from build123d import *

# Parameters (mm, degrees)
SKETCH_1_W          = 720
SKETCH_1_H          = 600
EXTRUDE_1_DEPTH     = 10
CUT_EXTRUDE_2_DEPTH = 469.72166581


with BuildPart() as part:
    # 草圖1 → 填料-伸長1 (new body)
    with BuildSketch(Plane.XY):
        Rectangle(SKETCH_1_W, SKETCH_1_H)
    extrude(amount=EXTRUDE_1_DEPTH)

    # 草圖2 → 除料-伸長2 (cut, through all)
    with BuildSketch(Plane.XY.offset(10)):
        with BuildLine():
            Line((-227, -52), (-195.192212959, -52))
            ThreePointArc((-195.192212959, -52), (-195.455703203, -51.000667501), (-195.714077164, -50))
            Line((-195.714077164, -50), (-225, -50))
            Line((-225, -50), (-225, 50))
            Line((-225, 50), (-195.714077164, 50))
            ThreePointArc((-195.714077164, 50), (-195.455703203, 51.000667501), (-195.192212959, 52))
            Line((-195.192212959, 52), (-227, 52))
            Line((-227, 52), (-227, -52))
        make_face()
        with BuildLine():
            Line((-225, -50), (-195.714077164, -50))
            ThreePointArc((-195.714077164, -50), (-202, 0), (-195.714077164, 50))
            Line((-195.714077164, 50), (-225, 50))
            Line((-225, 50), (-225, -50))
        make_face()
        with BuildLine():
            ThreePointArc((-193.64916731, 50), (-200, 0), (-193.64916731, -50))
            Line((-193.64916731, -50), (-125, -50))
            Line((-125, -50), (-125, 50))
            Line((-125, 50), (-193.64916731, 50))
        make_face()
        with BuildLine():
            ThreePointArc((-195.714077164, 50), (-202, 0), (-195.714077164, -50))
            Line((-195.714077164, -50), (-193.64916731, -50))
            ThreePointArc((-193.64916731, -50), (-200, 0), (-193.64916731, 50))
            Line((-193.64916731, 50), (-195.714077164, 50))
        make_face()
        with BuildLine():
            ThreePointArc((-193.64916731, 50), (-193.388030784, 51.000681851), (-193.121723273, 52))
            Line((-193.121723273, 52), (-195.192212959, 52))
            ThreePointArc((-195.192212959, 52), (-195.455703203, 51.000667501), (-195.714077164, 50))
            Line((-195.714077164, 50), (-193.64916731, 50))
        make_face()
        with BuildLine():
            ThreePointArc((-193.121723273, 52), (-141.421356237, 141.421356237), (-52, 193.121723273))
            Line((-52, 193.121723273), (-52, 195.192212959))
            ThreePointArc((-52, 195.192212959), (-142.8355698, 142.8355698), (-195.192212959, 52))
            Line((-195.192212959, 52), (-193.121723273, 52))
        make_face()
        with BuildLine():
            ThreePointArc((134.208828858, -148.283479378), (170.598797446, -104.384147791), (193.121723273, -52))
            Line((193.121723273, -52), (123, -52))
            Line((123, -52), (123, 52))
            Line((123, 52), (193.121723273, 52))
            ThreePointArc((193.121723273, 52), (141.421356237, 141.421356237), (52, 193.121723273))
            Line((52, 193.121723273), (52, 98))
            Line((52, 98), (-52, 98))
            Line((-52, 98), (-52, 193.121723273))
            ThreePointArc((-52, 193.121723273), (-141.421356237, 141.421356237), (-193.121723273, 52))
            Line((-193.121723273, 52), (-123, 52))
            Line((-123, 52), (-123, -52))
            Line((-123, -52), (-193.121723273, -52))
            ThreePointArc((-193.121723273, -52), (-170.598797446, -104.384147791), (-134.208828858, -148.283479378))
            Line((-134.208828858, -148.283479378), (-50, -224.499443206))
            ThreePointArc((-50, -224.499443206), (0, -230), (50, -224.499443206))
            Line((50, -224.499443206), (134.208828858, -148.283479378))
        make_face()
        with BuildLine():
            ThreePointArc((-193.64916731, -50), (-193.388030784, -51.000681851), (-193.121723273, -52))
            Line((-193.121723273, -52), (-123, -52))
            Line((-123, -52), (-123, 52))
            Line((-123, 52), (-193.121723273, 52))
            ThreePointArc((-193.121723273, 52), (-193.388030784, 51.000681851), (-193.64916731, 50))
            Line((-193.64916731, 50), (-125, 50))
            Line((-125, 50), (-125, -50))
            Line((-125, -50), (-193.64916731, -50))
        make_face()
        with BuildLine():
            Line((50, 100), (50, 193.64916731))
            ThreePointArc((50, 193.64916731), (25.200858902, 198.405939202), (8.18e-07, 200))
            ThreePointArc((8.18e-07, 200), (-25.200858091, 198.405939305), (-50, 193.64916731))
            Line((-50, 193.64916731), (-50, 100))
            Line((-50, 100), (50, 100))
        make_face()
        with BuildLine():
            Line((52, 98), (52, 193.121723273))
            ThreePointArc((52, 193.121723273), (51.000681851, 193.388030784), (50, 193.64916731))
            Line((50, 193.64916731), (50, 100))
            Line((50, 100), (-50, 100))
            Line((-50, 100), (-50, 193.64916731))
            ThreePointArc((-50, 193.64916731), (-51.000681851, 193.388030784), (-52, 193.121723273))
            Line((-52, 193.121723273), (-52, 98))
            Line((-52, 98), (52, 98))
        make_face()
        with BuildLine():
            ThreePointArc((-50, 195.714077164), (-39.236011871, 198.152808137), (-28.354893758, 200))
            Line((-28.354893758, 200), (-50, 200))
            Line((-50, 200), (-50, 195.714077164))
        make_face()
        with BuildLine():
            ThreePointArc((-28.354893758, 200), (-14.212670404, 201.499379652), (0, 202))
            Line((0, 202), (-52, 202))
            Line((-52, 202), (-52, 195.192212959))
            ThreePointArc((-52, 195.192212959), (-51.000667501, 195.455703203), (-50, 195.714077164))
            Line((-50, 195.714077164), (-50, 200))
            Line((-50, 200), (-28.354893758, 200))
        make_face()
        with BuildLine():
            Line((-52, 195.192212959), (-52, 193.121723273))
            ThreePointArc((-52, 193.121723273), (-51.000681851, 193.388030784), (-50, 193.64916731))
            Line((-50, 193.64916731), (-50, 195.714077164))
            ThreePointArc((-50, 195.714077164), (-51.000667501, 195.455703203), (-52, 195.192212959))
        make_face()
        with BuildLine():
            ThreePointArc((-50, 193.64916731), (-25.200858091, 198.405939305), (8.18e-07, 200))
            Line((8.18e-07, 200), (-28.354893758, 200))
            ThreePointArc((-28.354893758, 200), (-39.236011871, 198.152808137), (-50, 195.714077164))
            Line((-50, 195.714077164), (-50, 193.64916731))
        make_face()
        with BuildLine():
            ThreePointArc((28.354893758, 200), (14.212670404, 201.499379652), (0, 202))
            ThreePointArc((0, 202), (-14.212670404, 201.499379652), (-28.354893758, 200))
            Line((-28.354893758, 200), (8.18e-07, 200))
            Line((8.18e-07, 200), (28.354893758, 200))
        make_face()
        with BuildLine():
            ThreePointArc((50, 195.714077164), (51.000667501, 195.455703203), (52, 195.192212959))
            Line((52, 195.192212959), (52, 202))
            Line((52, 202), (0, 202))
            ThreePointArc((0, 202), (14.212670404, 201.499379652), (28.354893758, 200))
            Line((28.354893758, 200), (50, 200))
            Line((50, 200), (50, 195.714077164))
        make_face()
        with BuildLine():
            Line((50, 193.64916731), (50, 195.714077164))
            ThreePointArc((50, 195.714077164), (39.236011871, 198.152808137), (28.354893758, 200))
            Line((28.354893758, 200), (8.18e-07, 200))
            ThreePointArc((8.18e-07, 200), (25.200858902, 198.405939202), (50, 193.64916731))
        make_face()
        with BuildLine():
            ThreePointArc((28.354893758, 200), (39.236011871, 198.152808137), (50, 195.714077164))
            Line((50, 195.714077164), (50, 200))
            Line((50, 200), (28.354893758, 200))
        make_face()
        with BuildLine():
            Line((52, 193.121723273), (52, 195.192212959))
            ThreePointArc((52, 195.192212959), (51.000667501, 195.455703203), (50, 195.714077164))
            Line((50, 195.714077164), (50, 193.64916731))
            ThreePointArc((50, 193.64916731), (51.000681851, 193.388030784), (52, 193.121723273))
        make_face()
        with BuildLine():
            Line((193.121723273, 52), (195.192212959, 52))
            ThreePointArc((195.192212959, 52), (142.8355698, 142.8355698), (52, 195.192212959))
            Line((52, 195.192212959), (52, 193.121723273))
            ThreePointArc((52, 193.121723273), (141.421356237, 141.421356237), (193.121723273, 52))
        make_face()
        with BuildLine():
            Line((125, -50), (193.64916731, -50))
            ThreePointArc((193.64916731, -50), (200, 0), (193.64916731, 50))
            Line((193.64916731, 50), (125, 50))
            Line((125, 50), (125, -50))
        make_face()
        with BuildLine():
            ThreePointArc((193.121723273, -52), (193.388030784, -51.000681851), (193.64916731, -50))
            Line((193.64916731, -50), (125, -50))
            Line((125, -50), (125, 50))
            Line((125, 50), (193.64916731, 50))
            ThreePointArc((193.64916731, 50), (193.388030784, 51.000681851), (193.121723273, 52))
            Line((193.121723273, 52), (123, 52))
            Line((123, 52), (123, -52))
            Line((123, -52), (193.121723273, -52))
        make_face()
        with BuildLine():
            Line((195.714077164, -50), (225, -50))
            Line((225, -50), (225, 50))
            Line((225, 50), (195.714077164, 50))
            ThreePointArc((195.714077164, 50), (202, 0), (195.714077164, -50))
        make_face()
        with BuildLine():
            Line((193.64916731, -50), (195.714077164, -50))
            ThreePointArc((195.714077164, -50), (202, 0), (195.714077164, 50))
            Line((195.714077164, 50), (193.64916731, 50))
            ThreePointArc((193.64916731, 50), (200, 0), (193.64916731, -50))
        make_face()
        with BuildLine():
            Line((193.64916731, 50), (195.714077164, 50))
            ThreePointArc((195.714077164, 50), (195.455703203, 51.000667501), (195.192212959, 52))
            Line((195.192212959, 52), (193.121723273, 52))
            ThreePointArc((193.121723273, 52), (193.388030784, 51.000681851), (193.64916731, 50))
        make_face()
        with BuildLine():
            Line((225, 50), (225, -50))
            Line((225, -50), (195.714077164, -50))
            ThreePointArc((195.714077164, -50), (195.455703203, -51.000667501), (195.192212959, -52))
            Line((195.192212959, -52), (227, -52))
            Line((227, -52), (227, 52))
            Line((227, 52), (195.192212959, 52))
            ThreePointArc((195.192212959, 52), (195.455703203, 51.000667501), (195.714077164, 50))
            Line((195.714077164, 50), (225, 50))
        make_face()
        with BuildLine():
            ThreePointArc((195.192212959, -52), (195.455703203, -51.000667501), (195.714077164, -50))
            Line((195.714077164, -50), (193.64916731, -50))
            ThreePointArc((193.64916731, -50), (193.388030784, -51.000681851), (193.121723273, -52))
            Line((193.121723273, -52), (195.192212959, -52))
        make_face()
        with BuildLine():
            ThreePointArc((135.550917147, -149.766314172), (172.445114674, -105.198300486), (195.192212959, -52))
            Line((195.192212959, -52), (193.121723273, -52))
            ThreePointArc((193.121723273, -52), (170.598797446, -104.384147791), (134.208828858, -148.283479378))
            Line((134.208828858, -148.283479378), (50, -224.499443206))
            ThreePointArc((50, -224.499443206), (0, -230), (-50, -224.499443206))
            Line((-50, -224.499443206), (-134.208828858, -148.283479378))
            ThreePointArc((-134.208828858, -148.283479378), (-170.598797446, -104.384147791), (-193.121723273, -52))
            Line((-193.121723273, -52), (-195.192212959, -52))
            ThreePointArc((-195.192212959, -52), (-172.445114674, -105.198300486), (-135.550917147, -149.766314172))
            Line((-135.550917147, -149.766314172), (-50.951325963, -226.335950266))
            ThreePointArc((-50.951325963, -226.335950266), (0, -232), (50.951325963, -226.335950266))
            Line((50.951325963, -226.335950266), (135.550917147, -149.766314172))
        make_face()
        with BuildLine():
            ThreePointArc((-195.714077164, -50), (-195.455703203, -51.000667501), (-195.192212959, -52))
            Line((-195.192212959, -52), (-193.121723273, -52))
            ThreePointArc((-193.121723273, -52), (-193.388030784, -51.000681851), (-193.64916731, -50))
            Line((-193.64916731, -50), (-195.714077164, -50))
        make_face()
    extrude(amount=-CUT_EXTRUDE_2_DEPTH, mode=Mode.SUBTRACT)


solid = part.part
Source: CAD feature listing. Evaluate the final solid. Frame: model axes, mm. A direction names the side the tool comes from. Coordinates: 2 decimals unless noted, no trailing zeros. Loops run counter-clockwise (first coordinate to the right, second up) from the corner with the lowest first, then second, coordinate; pieces in that order, holes last. Notation, with made-up numbers: (53, 31) - (73, 31) arc R32 ccw to (73, 70) - close; hole circle Ø9 at (89.5, -8). An arc over 180 degrees is marked (long way). Return JSON: item names as keys, results as strings.
Q1. Material intervals for line 1 along X through (y, z) = (-16, 5); line 2 along Y through (x, z) = (199, 6.25); line 3 along X through (y, z) = (-128.5, 7), sorted ascending.
Results:
{"line 1": "-360 to -227, 227 to 360", "line 2": "-300 to -52, 52 to 300", "line 3": "-360 to -155.86, 155.86 to 360"}
Q2. Mould query, pull axis X, two halves, no side actions, for faces 3 (the flat face through (-5, 204, 10)), 4 (the cylindrical face through (143.882, 141.782, 5.07)). Classes: released by +X, released by -X, zero draft, split by the parting line, or undercut.
Results:
{"face 3": "zero draft", "face 4": "undercut"}
Q3. Section B-B, the plane x = 218.5. Return loops of the section in (y, z), plus the area to 3 significant figures.
Results:
{"outline": "(-300, 0) - (-52, 0) - (-52, 10) - (-300, 10) - close; (52, 0) - (300, 0) - (300, 10) - (52, 10) - close", "area": "4,960 mm2"}
Q4. Section A-A, the plane z = 7.5. Return loops of the section in (x, y), plus the area to 3 significant figures.
Results:
{"outline": "(-360, -300) - (360, -300) - (360, 300) - (-360, 300) - close; hole (-227, -52) - (-195.19, -52) arc R202 ccw to (-135.55, -149.77) - (-50.95, -226.34) arc R232 ccw to (50.95, -226.34) - (135.55, -149.77) arc R202 ccw to (195.19, -52) - (227, -52) - (227, 52) - (195.19, 52) arc R202 ccw to (52, 195.19) - (52, 202) - (-52, 202) - (-52, 195.19) arc R202 ccw to (-195.19, 52) - (-227, 52) - close", "area": "293,000 mm2"}
Q5. Access query for faces 1 (the flat face through (92.659, -188.587, 5.07)), 2 (the flat face through (-5, 204, 0)). Directions: +Z, -Z, +X, -X, +Y, -Y. A direction counts if a zero-diameter tool reaches every point of the face in a straight line with its end or side. Return the directions, or none.
Results:
{"face 1": "+Z, -Z", "face 2": "-Z, +X, -X, +Y, -Y"}
Q6. Section C-C, the plane y = -130. Return loops of the section in (x, z), plus the area to 3 significant figures.
Results:
{"outline": "(-360, 0) - (-154.61, 0) - (-154.61, 10) - (-360, 10) - close; (154.61, 0) - (360, 0) - (360, 10) - (154.61, 10) - close", "area": "4,110 mm2"}
